```python
from build123d import *

# Parameters (mm, degrees)
F0_R     = 16
F0_R_2   = 14.75
F1_DEPTH = 195
F0_R_3   = 17.5
F2_DEPTH = 165
F3_DEPTH = 35


with BuildPart() as f1:
    # F0 (on Top) → F1 (new body)
    with BuildSketch(Plane.XY):
        Circle(F0_R)
        Circle(F0_R_2, mode=Mode.SUBTRACT)
    extrude(amount=F1_DEPTH)

    # F0 (on Top) → F2 (join)
    with BuildSketch(Plane.XY):
        Circle(F0_R_3)
        Circle(F0_R, mode=Mode.SUBTRACT)
    extrude(amount=F2_DEPTH)

    # F0 (on Top) → F3 (cut)
    with BuildSketch(Plane.XY):
        Circle(F0_R)
        Circle(F0_R_2, mode=Mode.SUBTRACT)
    extrude(amount=F3_DEPTH, mode=Mode.SUBTRACT)


solid = f1.part
```
Here's how the part is built. I have some questions about the finished solid (model axes, mm). A direction names the side the tool comes from. Round coordinates to 2 decimals unless told otherwise and drop trailing zeros. Loops run counter-clockwise (first coordinate to the right, second up) from the corner with the lowest first, then second, coordinate; pieces in that order, holes last. Notation, with made-up numbers: (-3, 83) -> (31, 83) arc R11 cw to (31, 88) -> close; hole circle Ø8 at (-24, 16). An arc over 180 degrees is marked (long way). Answer as CSV lines item,"result". Start each with the question number.
1. I'm going to push flat-ended pins straight in: P1, Ø10, axis at y = 13.5, z = 127.5, coming from the -X side; P2, Ø12, axis at x = 7, z = 64, coming from the -Y side; P3, Ø6, axis at y = -9.5, z = 104, coming from the -X side. Where does each tip first touch, or does it pass through?
2. Imagine slicing it at A-A on y = 0. Write out the boundary of the cut face in (x, z).
3. For faces 4 (the face through (-13.887, -10.648, 81.345)), 5 (the face through (7.7, -14.2, 165)), 6 (the face through (-3.47, -15.62, 17.26)), which set-ups out of +Z, -Z, +X, -X, +Y, -Y let a thin tool reach every point of the face, with its end or its side?
4. Imagine slicing it at C-C on z = 44.5. Write out the boundary of the cut face in (x, y).
5. If we mould it in two halves opening along Y, with no side actions, what happens to faces 1 (the face through (-3.47, -15.62, 179.79)), 2 (the face through (14.07, 4.43, 113.88)), 3 (the face through (7.7, -14.2, 0))? For each: pulls with the +Y half, pulls with the -Y half, needs draft (parallel to the pull), parting line crosses it, or undercut.
6. I need wall thicknesses on probe 1 along Y at (x, z) = (0, 23); probe 2 along Y at (x, z) = (0, 67); probe 3 along X at (y, z) = (-11.5, 124). Which ranges of each line are inside material? Lowest first, please. Write a range as from..to.
Solution:
1,P1,"x = -15.3"
1,P2,"y = -17.47"
1,P3,"x = -16.25"
2,outline,"(-17.5, 0) -> (-16, 0) -> (-16, 35) -> (-14.75, 35) -> (-14.75, 195) -> (-16, 195) -> (-16, 165) -> (-17.5, 165) -> close; (14.75, 35) -> (16, 35) -> (16, 0) -> (17.5, 0) -> (17.5, 165) -> (16, 165) -> (16, 195) -> (14.75, 195) -> close"
3,face 4,"+Z, -Z"
3,face 5,"+Z"
3,face 6,"-Z"
4,outline,"circle Ø35 at (0, 0); hole circle Ø29.5 at (0, 0)"
5,face 1,"parting line crosses it"
5,face 2,"undercut"
5,face 3,"needs draft"
6,probe 1,"-17.5..-16, 16..17.5"
6,probe 2,"-17.5..-14.75, 14.75..17.5"
6,probe 3,"-13.19..-9.24, 9.24..13.19"
